Can you work these out from the model? Positions are in its coordinate system, mm. Face numbers are marked on the shaded views. A direction names the side the tool comes from. Coordinates: 2 decimals unless noted, no trailing zeros. Write each loop counter-clockwise with the first axis right and the second up, starting at its lowest first coordinate (ties: lowest second). Pieces come first, ordered by that corner, then holes. Notation, with made-up numbers: (38, 26.25) - (94, 26.25) arc R32 ccw to (94, 58.25) - close; hole circle Ø2 at (-29, 42.5). An arc over 180 degrees is marked (long way). One line per question, with ' | ' between items. Start each with the question number.
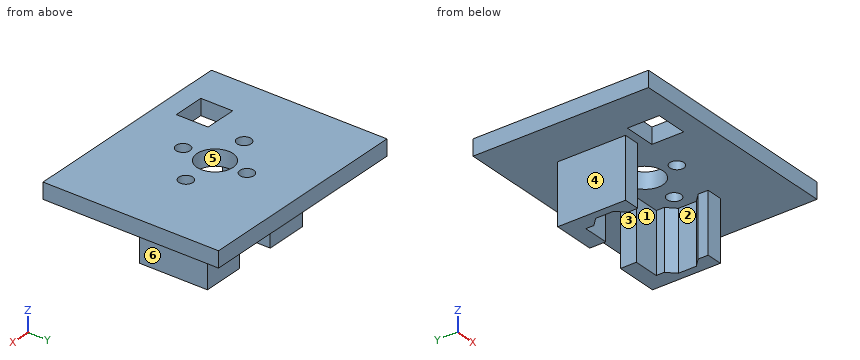
from build123d import *

# Parameters (mm, degrees)
SKETCH_W     = 55
SKETCH_H     = 44
SKETCH_R     = 1.75
SKETCH_R_2   = 4.5
SKETCH_W_2   = 8
SKETCH_H_2   = 8
PAD_DEPTH    = 4
PAD001_DEPTH = 15


with BuildPart() as part:
    # Sketch → Pad (new body)
    with BuildSketch(Plane.XY):
        Rectangle(SKETCH_W, SKETCH_H)
        with Locations((-9.5, 0)):
            Circle(SKETCH_R, mode=Mode.SUBTRACT)
        with Locations((0, 8)):
            Circle(SKETCH_R, mode=Mode.SUBTRACT)
        with Locations((9.5, 0)):
            Circle(SKETCH_R, mode=Mode.SUBTRACT)
        with Locations((0, -8)):
            Circle(SKETCH_R, mode=Mode.SUBTRACT)
        Circle(SKETCH_R_2, mode=Mode.SUBTRACT)
        with Locations((-13.5, -13)):
            Rectangle(SKETCH_W_2, SKETCH_H_2, mode=Mode.SUBTRACT)
    extrude(amount=PAD_DEPTH)

    # Sketch001 (on Face14 of Pad) → Pad001 (join)
    with BuildSketch(Plane(origin=(0, 0, 0), x_dir=(1, 0, 0), z_dir=(0, 0, -1))):
        Polygon((-15.5, 7), (-11.5, 7), (-11.5, 4.5), (-13.5, 2.5), (-13.5, -2), (-11.5, -4), (-11.5, -6), (-5, -6), (-5, -10), (-15.5, -10), align=None)
        Polygon((11.5, 7), (15.5, 7), (15.5, -10), (5, -10), (5, -6), (11.5, -6), (11.5, -4), (13.5, -2), (13.5, 2.5), (11.5, 4.5), align=None)
    extrude(amount=PAD001_DEPTH)


solid = part.part
(1) If we section it at C-C on x = 9.5: List the corners of the cut face in (y, z) for me, plus the area to 3 significant figures.
(2) If we section it at D-D on y = 0: List the corners of the cut face in (x, z) for me.
(3) If we section it at A-A on y = 8: List the corners of the cut face in (x, z) for me.
(4) If we section it at B-B on z = -10.75: List the corners of the cut face in (x, y) for me, plus the area to 3 significant figures.
(5) Which directions (+Z, -Z, +X, -X, +Y, -Y) give clear straight access to the entire face, cutting with the end or side of a thin tool? Please do the marked faces 4, 5 and 6.
(6) I'm going to push flat-ended pins straight in: pin 1 (2 mm diameter, centred on x = 2, y = -12, fed in from -Z); pin 2 (3 mm diameter, centred on y = -6, z = -5.5, fed in from -X); pin 3 (1.3 mm diameter, centred on y = 0.5, z = -10, fed in from +X). Where does each tip first touch, or does it pass through?
(7) If we mould it in two halves opening along Y, with no side actions, what happens to the marked faces 1, 2 and 3? For each: +Y half, -Y half, draft (parallel to the pull), parting line (faces both ways), or undercut.
(8) If I drill on probe 1 along Y at (x, z) = (0, 2.45); probe 2 along Y at (x, z) = (-12, 2); probe 3 along X at (y, z) = (7, -0.5), over which ranges is the centre line in solid material (lowest first)?
Values:
1) outline: (-22, 0) - (-1.75, 0) - (-1.75, 4) - (-22, 4) - close; (1.75, 0) - (6, 0) - (6, -15) - (10, -15) - (10, 0) - (22, 0) - (22, 4) - (1.75, 4) - close | area: 222 mm2
2) outline: (-27.5, 0) - (-15.5, 0) - (-15.5, -15) - (-13.5, -15) - (-13.5, 0) - (-11.25, 0) - (-11.25, 4) - (-27.5, 4) - close; (-7.75, 0) - (-4.5, 0) - (-4.5, 4) - (-7.75, 4) - close; (4.5, 0) - (7.75, 0) - (7.75, 4) - (4.5, 4) - close; (11.25, 0) - (13.5, 0) - (13.5, -15) - (15.5, -15) - (15.5, 0) - (27.5, 0) - (27.5, 4) - (11.25, 4) - close
3) outline: (-27.5, 0) - (-15.5, 0) - (-15.5, -15) - (-5, -15) - (-5, 0) - (-1.75, 0) - (-1.75, 4) - (-27.5, 4) - close; (1.75, 0) - (5, 0) - (5, -15) - (15.5, -15) - (15.5, 0) - (27.5, 0) - (27.5, 4) - (1.75, 4) - close
4) outline: (-15.5, -7) - (-11.5, -7) - (-11.5, -4.5) - (-13.5, -2.5) - (-13.5, 2) - (-11.5, 4) - (-11.5, 6) - (-5, 6) - (-5, 10) - (-15.5, 10) - close; (5, 6) - (11.5, 6) - (11.5, 4) - (13.5, 2) - (13.5, -2.5) - (11.5, -4.5) - (11.5, -7) - (15.5, -7) - (15.5, 10) - (5, 10) - close | area: 162 mm2
5) face 4: -Z, -X, +Y, -Y | face 5: +Z, -Z | face 6: -Z, +X, +Y, -Y
6) pin 1: z = 0 | pin 2: x = -15.5 | pin 3: x = 15.5
7) face 1: -Y half | face 2: undercut | face 3: draft
8) probe 1: -22 to -9.75, -6.25 to -4.5, 4.5 to 6.25, 9.75 to 22 | probe 2: -22 to -17, -9 to 22 | probe 3: -15.5 to -5, 5 to 15.5
